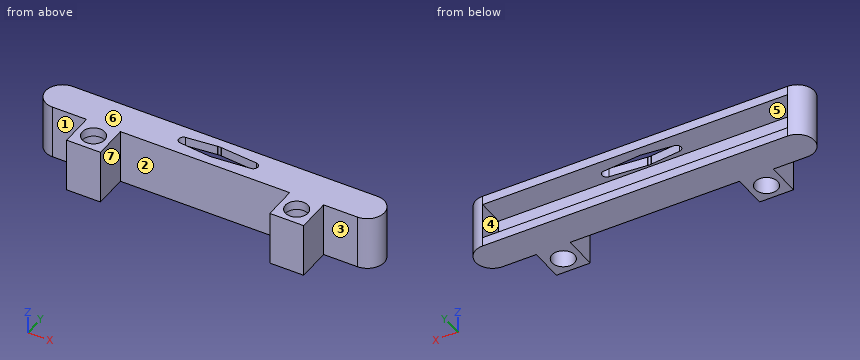
```python
from build123d import *

# Parameters (mm, degrees)
SKETCH1_R           = 5
BOSS_EXTRUDE1_DEPTH = 4
SKETCH1_4_R         = 5
BOSS_EXTRUDE2_DEPTH = 20
SKETCH2_W           = 135
SKETCH2_H           = 16
CUT_EXTRUDE1_DEPTH  = 12


with BuildPart() as part:
    # Sketch1 → Boss-Extrude1 (new body)
    with BuildSketch(Plane.XY):
        with BuildLine():
            Line((52.5, -7.5), (67.5, -7.5))
            ThreePointArc((67.5, -7.5), (75, 0), (67.5, 7.5))
            Line((67.5, 7.5), (-67.5, 7.5))
            ThreePointArc((-67.5, 7.5), (-75, 0), (-67.5, -7.5))
            Line((-67.5, -7.5), (-52.5, -7.5))
            Line((-52.5, -7.5), (-52.5, -22.5))
            Line((-52.5, -22.5), (-37.5, -22.5))
            Line((-37.5, -22.5), (-37.5, -7.5))
            Line((-37.5, -7.5), (37.5, -7.5))
            Line((37.5, -7.5), (37.5, -22.5))
            Line((37.5, -22.5), (52.5, -22.5))
            Line((52.5, -22.5), (52.5, -7.5))
        make_face()
        with BuildLine():
            Line((-14.211482552, 1.988787352), (-0.965077795, 3.3973761))
            ThreePointArc((-0.965077795, 3.3973761), (-0.860540111, 3.407937274), (-0.755897232, 3.417399505))
            ThreePointArc((-0.755897232, 3.417399505), (-0.049360306, 3.49965192), (0.65921534, 3.437358744))
            ThreePointArc((0.65921534, 3.437358744), (0.81309385, 3.427430851), (0.966800983, 3.415131426))
            Line((0.966800983, 3.415131426), (17.174893203, 1.992338417))
            ThreePointArc((17.174893203, 1.992338417), (19, 0), (17.174893203, -1.992338417))
            Line((17.174893203, -1.992338417), (0.966800983, -3.415131426))
            ThreePointArc((0.966800983, -3.415131426), (0.81309385, -3.427430851), (0.65921534, -3.437358744))
            ThreePointArc((0.65921534, -3.437358744), (-0.049360306, -3.49965192), (-0.755897232, -3.417399505))
            ThreePointArc((-0.755897232, -3.417399505), (-0.860540111, -3.407937274), (-0.965077795, -3.3973761))
            Line((-0.965077795, -3.3973761), (-14.211482552, -1.988787352))
            ThreePointArc((-14.211482552, -1.988787352), (-16, 0), (-14.211482552, 1.988787352))
        make_face(mode=Mode.SUBTRACT)
        with Locations((45, -15)):
            Circle(SKETCH1_R, mode=Mode.SUBTRACT)
        with Locations((-45, -15)):
            Circle(SKETCH1_R, mode=Mode.SUBTRACT)
    extrude(amount=BOSS_EXTRUDE1_DEPTH)

    # Sketch1_4 → Boss-Extrude2 (add)
    with BuildSketch(Plane.XY):
        with BuildLine():
            Line((52.5, -7.5), (67.5, -7.5))
            ThreePointArc((67.5, -7.5), (75, 0), (67.5, 7.5))
            Line((67.5, 7.5), (-67.5, 7.5))
            ThreePointArc((-67.5, 7.5), (-75, 0), (-67.5, -7.5))
            Line((-67.5, -7.5), (-52.5, -7.5))
            Line((-52.5, -7.5), (-52.5, -22.5))
            Line((-52.5, -22.5), (-37.5, -22.5))
            Line((-37.5, -22.5), (-37.5, -7.5))
            Line((-37.5, -7.5), (37.5, -7.5))
            Line((37.5, -7.5), (37.5, -22.5))
            Line((37.5, -22.5), (52.5, -22.5))
            Line((52.5, -22.5), (52.5, -7.5))
        make_face()
        with Locations((-45, -15)):
            Circle(SKETCH1_4_R, mode=Mode.SUBTRACT)
        with Locations((45, -15)):
            Circle(SKETCH1_4_R, mode=Mode.SUBTRACT)
    extrude(amount=-BOSS_EXTRUDE2_DEPTH)

    # Sketch2 → Cut-Extrude1 (cut)
    with BuildSketch(Plane(origin=(0, 7.5, 0), x_dir=(1, 0, 0), z_dir=(0, 1, 0))):
        with Locations((0, 8)):
            Rectangle(SKETCH2_W, SKETCH2_H)
    extrude(amount=-CUT_EXTRUDE1_DEPTH, mode=Mode.SUBTRACT)


solid = part.part
```
Can you work these out from the model? Positions are in its coordinate system, mm. Face numbers are marked on the shaded views. A direction names the side the tool comes from. Give positions to 0.01 mm unless a question says otherwise; leave off trailing zeros. Loops run counter-clockwise (first coordinate to the right, second up) from the corner with the lowest first, then second, coordinate; pieces in that order, holes last. Notation, with made-up numbers: M 72.25,-27 L 125.25,-27 A25 ccw 125.25,-5 Z; hole C -39,81 d8. An arc over 180 degrees is marked long. Use CSV: the item, a comma, the result in double quotes. Start each with the question number.
1. If we mould it in two halves opening along Z, with no side actions, what happens to the marked faces 4, 5, 6 and 7? For each: released by +Z, released by -Z, zero draft, split by the parting line, or undercut.
2. On a 3-axis mill with a long thin cutter (end or side, diameter ignored), from which of +Z, -Z, +X, -X, +Y, -Y can I reach the whole of each face in a straight line? I mean the marked faces 1, 2 and 3. Say none if no direction works.
3. Imagine slicing it at C-C, the plane x = 45. Write out the boundary of the cut face in (y, z).
4. If I drill on L1, parallel to Y at x = 45, z = 1.6; L2, parallel to Y at x = -45, z = -7.5; L3, parallel to X at y = -16, z = -1, over which ranges is the centre line in solid material (lowest first)?
5. Imagine slicing it at A-A, the plane z = -17.25. Write out the boundary of the cut face in (x, y), plus the area to 3 significant figures.
6. Imagine slicing it at D-D, the plane y = -15. Write out the boundary of the cut face in (x, z), plus the area to 3 significant figures.
7. For P1, Ø4.5, axis at x = -59.5, z = -8.5, coming from the -Y side; P2, Ø6, axis at y = -14.5, z = -8, coming from the -X side; P3, Ø6, axis at x = 45, y = -15, coming from the -Z side; P4, Ø7.5, axis at y = -15, z = -7, coming from the +X side, each with a flat end and sliding along its axis, tell me the tip position at first contact or that it passes through.
8. Imagine slicing it at B-B, the plane z = 2.5. Write out the boundary of the cut face in (x, y).
Response values:
1,face 4,"undercut"
1,face 5,"undercut"
1,face 6,"released by +Z"
1,face 7,"zero draft"
2,face 1,"+Z, -Z, -X, -Y"
2,face 2,"+Z, -Z, -Y"
2,face 3,"+Z, -Z, +X, -Y"
3,outline,"M -22.5,-20 L -20,-20 L -20,4 L -22.5,4 Z; M -10,-20 L 7.5,-20 L 7.5,-16 L -4.5,-16 L -4.5,0 L 7.5,0 L 7.5,4 L -10,4 Z"
4,L1,"-22.5 to -20, -10 to 7.5"
4,L2,"-22.5 to -20, -10 to -4.5"
4,L3,"-52.5 to -49.9, -40.1 to -37.5, 37.5 to 40.1, 49.9 to 52.5"
5,outline,"M -67.5,-7.5 L -52.5,-7.5 L -52.5,-22.5 L -37.5,-22.5 L -37.5,-7.5 L 37.5,-7.5 L 37.5,-22.5 L 52.5,-22.5 L 52.5,-7.5 L 67.5,-7.5 A7.5 ccw 67.5,7.5 L -67.5,7.5 A7.5 ccw Z; hole C -45,-15 d10; hole C 45,-15 d10"
5,area,"2,490 mm^2"
6,outline,"M -52.5,-20 L -50,-20 L -50,4 L -52.5,4 Z; M -40,-20 L -37.5,-20 L -37.5,4 L -40,4 Z; M 37.5,-20 L 40,-20 L 40,4 L 37.5,4 Z; M 50,-20 L 52.5,-20 L 52.5,4 L 50,4 Z"
6,area,"240 mm^2"
7,P1,"y = -7.5"
7,P2,"x = -52.5"
7,P3,"through"
7,P4,"x = 52.5"
8,outline,"M -67.5,-7.5 L -52.5,-7.5 L -52.5,-22.5 L -37.5,-22.5 L -37.5,-7.5 L 37.5,-7.5 L 37.5,-22.5 L 52.5,-22.5 L 52.5,-7.5 L 67.5,-7.5 A7.5 ccw 67.5,7.5 L -67.5,7.5 A7.5 ccw Z; hole C -45,-15 d10; hole M -14.21,-1.99 L -0.97,-3.4 A10 ccw -0.76,-3.42 A3.5 ccw 0.66,-3.44 A10 ccw 0.97,-3.42 L 17.17,-1.99 A2 ccw 17.17,1.99 L 0.97,3.42 A10 ccw 0.66,3.44 A3.5 ccw -0.76,3.42 A10 ccw -0.97,3.4 L -14.21,1.99 A2 ccw Z; hole C 45,-15 d10"
